from build123d import *

# Parameters (mm, degrees)
F1_DEPTH = 3
F3_DEPTH = 3


with BuildPart() as f1:
    # F0 (on Front) → F1 (new body)
    with BuildSketch(Plane.XZ):
        with BuildLine():
            Line((28, -8), (32.5, -8))
            Line((32.5, -8), (32.5, 16))
            Line((32.5, 16), (18, 16))
            Line((18, 16), (18, 19))
            Line((18, 19), (10, 19))
            Line((10, 19), (10, 16))
            Line((10, 16), (0, 16))
            Line((0, 16), (-10, 16))
            Line((-10, 16), (-10, 19))
            Line((-10, 19), (-18, 19))
            Line((-18, 19), (-18, 16))
            Line((-18, 16), (-32.5, 16))
            Line((-32.5, 16), (-32.5, -8))
            Line((-32.5, -8), (-28, -8))
            Line((-28, -8), (-28, -11))
            Line((-28, -11), (-20, -11))
            Line((-20, -11), (-20, -8))
            Line((-20, -8), (-6, -8))
            ThreePointArc((-6, -8), (-4.472136, 8.944272), (10, 0))
            ThreePointArc((10, 0), (8.944272, -4.472136), (6, -8))
            Line((6, -8), (20, -8))
            Line((20, -8), (20, -11))
            Line((20, -11), (28, -11))
            Line((28, -11), (28, -8))
        make_face()
    extrude(amount=F1_DEPTH)

    # F2 (on face) → F3 (cut, through all)
    with BuildSketch(Plane(origin=(0, 0, 0), x_dir=(-1, 0, 0), z_dir=(0, 1, 0))):
        Polygon((13, -5), (13, -8), (16, -8), (16, -5), (17.5, -5), (17.5, -2.5), (16, -2.5), (16, -0.5), (13, -0.5), (13, -2.5), (11.5, -2.5), (11.5, -5), align=None)
        Polygon((-11.5, -2.5), (-13, -2.5), (-13, -0.5), (-16, -0.5), (-16, -2.5), (-17.5, -2.5), (-17.5, -5), (-16, -5), (-16, -8), (-13, -8), (-13, -5), (-11.5, -5), align=None)
        Polygon((26, 13), (26, 16), (23, 16), (23, 13), (21.5, 13), (21.5, 10.5), (23, 10.5), (23, 7.5), (26, 7.5), (26, 10.5), (27.5, 10.5), (27.5, 13), align=None)
        Polygon((-23, 10.5), (-21.5, 10.5), (-21.5, 13), (-23, 13), (-23, 16), (-26, 16), (-26, 13), (-27.5, 13), (-27.5, 10.5), (-26, 10.5), (-26, 7.5), (-23, 7.5), align=None)
    extrude(amount=-F3_DEPTH, mode=Mode.SUBTRACT)


solid = f1.part
Build history of the part. All positions in model axes, mm. A direction names the side the tool comes from. Coordinates: 2 decimals unless noted, no trailing zeros. Order: outer loops, then holes, each group sorted by start corner. A loop starts at its lowest first (then second) coordinate and runs counter-clockwise, first axis right, second up. Notation, with made-up numbers: (39, 40) - (95, 40) arc R30 ccw to (95, 76) - close; hole circle Ø3 at (30, -2). An arc over 180 degrees is marked (long way). Put each result on its own line as item: value.
1. Saw through at B-B (x = -15). Write the cut outline in (y, z).
Answer sheet:
outline: (-3, -0.5) - (0, -0.5) - (0, 19) - (-3, 19) - close
2. Drop flat-ended pins along their axis: P1, Ø1.5, axis at y = -1, z = 18, coming from the -X side; P2, Ø0.9, axis at x = 18.5, y = -1.5, coming from the -Z side; P3, Ø1.5, axis at x = 14, y = -1.5, coming from the -Z side. Give the stop position or say it passes through.
Answer sheet:
P1: stops at x = -18
P2: stops at z = -8
P3: stops at z = -0.5
3. Saw through at C-C (z = 1). Write the cut outline in (x, y).
Answer sheet:
outline: (-32.5, -3) - (-9.95, -3) - (-9.95, 0) - (-32.5, 0) - close; (9.95, -3) - (32.5, -3) - (32.5, 0) - (9.95, 0) - close
4. Saw through at D-D (x = 19). Write the cut outline in (y, z), and give its area (3 significant figures).
Answer sheet:
outline: (-3, -8) - (0, -8) - (0, 16) - (-3, 16) - close
area: 72.0 mm^2
5. Probe line 1 along X through (y, z) = (-2.1, 12); line 2 along Z through (x, y) = (-17, -2.4); line 3 along X through (y, z) = (-0.9, 0). List the from-to ranges inside material, lowest first. Write a range as [from, to].
Answer sheet:
line 1: x = [-32.5, -27.5], [-21.5, 21.5], [27.5, 32.5]
line 2: z = [-8, -5], [-2.5, 19]
line 3: x = [-32.5, -10], [10, 32.5]
6. Pull direction X, two halves, no side cores. Call faces 1 (the face through (-24, -1, -11)), 2 (the face through (-23, -1, 15)), 3 (the face through (-18, -1, 18)): pulls with the +X half, pulls with the -X half, needs draft (parallel to the pull), parting line crosses it, or undercut.
Answer sheet:
face 1: needs draft
face 2: undercut
face 3: pulls with the -X half
7. Saw through at A-A (z = -8.75). Write the cut outline in (x, y).
Answer sheet:
outline: (-28, -3) - (-20, -3) - (-20, 0) - (-28, 0) - close; (20, -3) - (28, -3) - (28, 0) - (20, 0) - close
8. Tool access for faces 4 (the face through (-17, -1, -2.5)), 5 (the face through (18, -1, -8)), 6 (the face through (10, -1, 18)), 7 (the face through (-30, -1, -8)): list every direction of +Z, -Z, +X, -X, +Y, -Y with a clear straight run to the whole face (end or side of a thin tool).
Answer sheet:
face 4: +Y, -Y
face 5: -Z, +Y, -Y
face 6: +Z, +Y, -Y
face 7: -Z, -X, +Y, -Y
